Verification items for the finished model (mm, model axes). Give positions to 0.01 mm unless a question says otherwise; leave off trailing zeros. Write each loop counter-clockwise with the first axis right and the second up, starting at its lowest first coordinate (ties: lowest second). Pieces come first, ordered by that corner, then holes. Notation, with made-up numbers: (-9, -29) - (8, -29) arc R17 ccw to (8, 2) - close; hole circle Ø9 at (22.5, -16). An arc over 180 degrees is marked (long way). Answer as a JSON object with one key per item and string values. Group by question number.
Item 1: Sectioned sample at A-A, the plane z = 0. Record the boundary of the cut face in (x, y), and give its area (3 significant figures).
Item 2: Sectioned sample at C-C, the plane z = 22. Record the boundary of the cut face in (x, y).
Item 3: Scan lines: line 1 along Y through (x, z) = (2.55, 0); line 2 along Y through (x, z) = (1.3, 0); line 3 along Z through (x, y) = (0.55, 12). Record each from-to range of solid material in increasing order. Write a range as [from, to].
Item 4: Draft check along Z on faces 1 (the face through (3.97, -15.62, 3.47)), 2 (the face through (3.042, 29.699, -38.833)), 3 (the face through (3.04, 6.74, 27.91)), 4 (the face through (6, 19, 1)). Enter one of: +Z half, -Z half, draft (parallel to the pull), parting line (faces both ways), or undercut.
Item 5: Sectioned sample at B-B, the plane y = 5.5. Record the boundary of the cut face in (x, z).
Item 6: Sectioned sample at D-D, the plane x = 3.15. Record the boundary of the cut face in (y, z), and give its area (3 significant figures).
Item 7: Go/stop test with flat-tipped pins: pin 1 (12 mm diameter, centred on y = 6.5, z = -10.5, fed in from -X); pin 2 (1 mm diameter, centred on x = 2, z = 15, fed in from -Y) (3 decimals); pin 3 (1 mm diameter, centred on x = 5, z = -1.5, fed in from -Y) (3 decimals). Record where each tip stops, or that it passes through.
```python
from build123d import *

# Parameters (mm, degrees)
SKETCH1_R           = 20
SKETCH1_R_2         = 15
BOSS_EXTRUDE1_DEPTH = 2
SKETCH2_R           = 20
SKETCH2_R_2         = 16
BOSS_EXTRUDE2_DEPTH = 4
SKETCH3_R           = 2
BOSS_EXTRUDE3_DEPTH = 6
SKETCH4_R           = 2.4
CUT_EXTRUDE1_DEPTH  = 6
SKETCH5_R           = 2
SKETCH5_R_2         = 1.55
BOSS_EXTRUDE4_DEPTH = 6


with BuildPart() as part:
    # Sketch1 → Boss-Extrude1 (new body)
    with BuildSketch(Plane(origin=(0, 0, 0), x_dir=(0, 0, -1), z_dir=(1, 0, 0))):
        Circle(SKETCH1_R)
        Circle(SKETCH1_R_2, mode=Mode.SUBTRACT)
    extrude(amount=BOSS_EXTRUDE1_DEPTH)

    # Sketch2 → Boss-Extrude2 (add)
    with BuildSketch(Plane(origin=(2, 0, 0), x_dir=(0, 0, -1), z_dir=(1, 0, 0))):
        Circle(SKETCH2_R)
        Circle(SKETCH2_R_2, mode=Mode.SUBTRACT)
    extrude(amount=BOSS_EXTRUDE2_DEPTH)

    # Sketch3 → Boss-Extrude3 (add)
    with BuildSketch(Plane(origin=(6, 0, 0), x_dir=(0, 0, -1), z_dir=(1, 0, 0))):
        with BuildLine():
            Line((-38.608830959, 23.677807584), (-16.909895057, -10.679674581))
            ThreePointArc((-16.909895057, -10.679674581), (0, 20), (16.909895057, -10.679674581))
            Line((16.909895057, -10.679674581), (38.608830959, 23.677807584))
            ThreePointArc((38.608830959, 23.677807584), (38.790546744, 29.777964933), (33.535862442, 32.881709959))
            Line((33.535862442, 32.881709959), (-33.535862442, 32.881709959))
            ThreePointArc((-33.535862442, 32.881709959), (-38.790546744, 29.777964933), (-38.608830959, 23.677807584))
        make_face()
        with Locations((-33.535862442, 26.881709959)):
            Circle(SKETCH3_R, mode=Mode.SUBTRACT)
        with Locations((33.535862442, 26.881709959)):
            Circle(SKETCH3_R, mode=Mode.SUBTRACT)
    extrude(amount=-BOSS_EXTRUDE3_DEPTH)

    # Sketch4 → Cut-Extrude1 (cut)
    with BuildSketch(Plane(origin=(6, 0, 0), x_dir=(0, 0, -1), z_dir=(1, 0, 0))):
        with Locations((-22.856187861, 9.971814902)):
            Circle(SKETCH4_R)
        with Locations((22.856187861, 9.971814902)):
            Circle(SKETCH4_R)
        with Locations((0, 26.881709959)):
            Circle(SKETCH4_R)
    extrude(amount=-CUT_EXTRUDE1_DEPTH, mode=Mode.SUBTRACT)

    # Sketch5 → Boss-Extrude4 (add)
    with BuildSketch(Plane(origin=(0, 0, 0), x_dir=(0, 0, -1), z_dir=(1, 0, 0))):
        with Locations((33.535862442, 26.881709959)):
            Circle(SKETCH5_R)
        with Locations((33.535862442, 26.881709959)):
            Circle(SKETCH5_R_2, mode=Mode.SUBTRACT)
        with Locations((-33.535862442, 26.881709959)):
            Circle(SKETCH5_R)
        with Locations((-33.535862442, 26.881709959)):
            Circle(SKETCH5_R_2, mode=Mode.SUBTRACT)
    extrude(amount=BOSS_EXTRUDE4_DEPTH)


solid = part.part
```
Geometry check:
{
 "1": {"outline": "(0, -20) - (6, -20) - (6, -16) - (2, -16) - (2, -15) - (0, -15) - close; (0, 15) - (2, 15) - (2, 16) - (6, 16) - (6, 24.48) - (0, 24.48) - close; (0, 29.28) - (6, 29.28) - (6, 32.88) - (0, 32.88) - close", "area": "100 mm^2"},
 "2": {"outline": "(0, -2.62) - (6, -2.62) - (6, 7.73) - (0, 7.73) - close; (0, 12.21) - (6, 12.21) - (6, 32.88) - (0, 32.88) - close"},
 "3": {"line 1": "[-20, -16], [16, 24.48], [29.28, 32.88]", "line 2": "[-20, -15], [15, 24.48], [29.28, 32.88]", "line 3": "[-31.23, -24.14], [-21.57, -9], [9, 21.57], [24.14, 31.23]"},
 "4": {"face 1": "undercut", "face 2": "-Z half", "face 3": "+Z half", "face 4": "draft"},
 "5": {"outline": "(0, -27.13) - (6, -27.13) - (6, -15.02) - (2, -15.02) - (2, -13.96) - (0, -13.96) - close; (0, 13.96) - (2, 13.96) - (2, 15.02) - (6, 15.02) - (6, 27.13) - (0, 27.13) - close"},
 "6": {"outline": "(-10.68, -16.91) - (23.68, -38.61) arc R6 ccw to (32.88, -33.54) - (32.88, 33.54) arc R6 ccw to (23.68, 38.61) - (-10.68, 16.91) arc R20 ccw to start; hole circle Ø32 at (0, 0); hole circle Ø4.8 at (9.97, -22.86); hole circle Ø4.8 at (9.97, 22.86); hole circle Ø4.8 at (26.88, 0); hole circle Ø3.1 at (26.88, -33.54); hole circle Ø3.1 at (26.88, 33.54)", "area": "1,970 mm^2"},
 "7": {"pin 1": "x = 0", "pin 2": "y = -13.775", "pin 3": "y = -19.975"}
}
